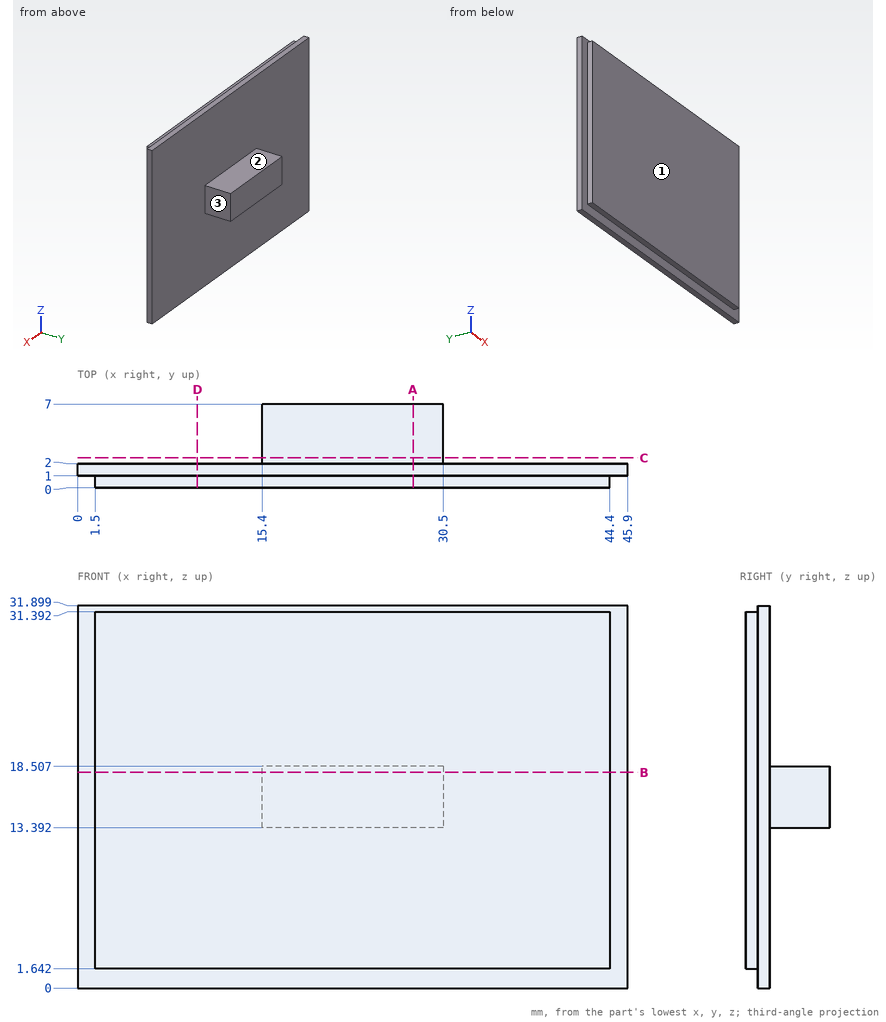
Geometry: see drawing. Coordinates: mm, zero at the bounding-box minimum. A direction names the side the tool comes from. Coordinates: 2 decimals unless noted, no trailing zeros. Loops run counter-clockwise (first coordinate to the right, second up) from the corner with the lowest first, then second, coordinate; pieces in that order, holes last.
Q1. Cut plane A-A (x = 28). Output: boundary loops of the cut face in (y, z), then the cut area to 3 significant figures.
Q2. Contact query for flat-ended pins moving along their axis: pin 1 (4 mm diameter, centred on x = 17.5, z = 26, fed in from -Y); pin 2 (2.5 mm diameter, centred on y = 4.5, z = 15, fed in from -X); pin 3 (0.5 mm diameter, centred on x = 21.5, y = 0.5, fed in from -Z); pin 4 (0.8 mm diameter, centred on y = 0.5, z = 10.5, fed in from +X). Output: stop coordinate, or through.
Q3. Material intervals for line 1 (Y direction, x = 39, z = 28); line 2 (Z direction, x = 27, y = 6.75); line 3 (X direction, y = 3.5, z = 16), sorted ascending.
Q4. Cut plane B-B (z = 18). Output: boundary loops of the cut face in (x, y).
Q5. Set-up query: the marked faces 1, 2 and 3. Return all of +Z, -Z, +X, -X, +Y, -Y with unobstructed straight access to the full face (end or side cutting, diameter ignored); none if empty.
Q6. Cut plane D-D (x = 10). Output: boundary loops of the cut face in (y, z).
Q7. Cut plane C-C (y = 2.5). Output: boundary loops of the cut face in (x, z).
Working result:
1. outline: (0, 1.64) - (1, 1.64) - (1, 0) - (2, 0) - (2, 13.39) - (7, 13.39) - (7, 18.51) - (2, 18.51) - (2, 31.9) - (1, 31.9) - (1, 31.39) - (0, 31.39) - close
1. area: 87.2 mm2
2. pin 1: stops at y = 0
2. pin 2: stops at x = 15.4
2. pin 3: stops at z = 1.64
2. pin 4: stops at x = 44.4
3. line 1: y = 0 to 2
3. line 2: z = 13.39 to 18.51
3. line 3: x = 15.4 to 30.5
4. outline: (0, 1) - (1.5, 1) - (1.5, 0) - (44.4, 0) - (44.4, 1) - (45.9, 1) - (45.9, 2) - (30.5, 2) - (30.5, 7) - (15.4, 7) - (15.4, 2) - (0, 2) - close
5. face 1: +Z, -Z, +X, -X, -Y
5. face 2: +Z, +X, -X, +Y
5. face 3: +Z, -Z, +X, +Y
6. outline: (0, 1.64) - (1, 1.64) - (1, 0) - (2, 0) - (2, 31.9) - (1, 31.9) - (1, 31.39) - (0, 31.39) - close
7. outline: (15.4, 13.39) - (30.5, 13.39) - (30.5, 18.51) - (15.4, 18.51) - close
